Geometry check sheet. Reference: the model listing, model coordinates, mm. A direction names the side the tool comes from. Round coordinates to 2 decimals unless told otherwise and drop trailing zeros. Order: outer loops, then holes, each group sorted by start corner. A loop starts at its lowest first (then second) coordinate and runs counter-clockwise, first axis right, second up. Notation, with made-up numbers: (-16.75, -28) - (-1.75, -28) arc R15 cw to (-1.75, -15) - close; hole circle Ø3 at (-29.5, -21.75). An arc over 180 degrees is marked (long way). One line per question, with ' | ' between items. Start each with the question number.
Q1. Sectioned sample at B-B, the plane z = 67. Enter the section's corners in (x, y).
Q2. Tool access check on faces 1 (the face through (0, -356, -508)), 2 (the face through (0, 2, 584.2)). Record the directions out of +Z, -Z, +X, -X, +Y, -Y that give a thin tool (end or side, any length) a straight path to the whole face; none if there is none.
Q3. Material ranges on line 1 along Y through (x, z) = (-6, -224.5); line 2 along Z through (x, y) = (-5.25, -388.5); line 3 along Y through (x, z) = (-1, -358), recorded low to high.
Q4. Sectioned sample at C-C, the plane y = -225. Enter the section's corners in (x, z).
Q5. Sectioned sample at A-A, the plane x = -1.75. Enter the section's corners in (y, z).
Q6. Gauge pin test, flat ends, axial feed: P1, Ø12.5, axis at x = -5, z = 147, coming from the -Y side; P2, Ø12.5, axis at x = 6, y = -336, coming from the +Z side. Record the tip position at first contact, or that the pin passes through.
```python
from build123d import *

# Parameters (mm, degrees)
F0_W     = 355.6
F0_H     = 254
F1_DEPTH = 12.7
F3_DEPTH = 25.401


with BuildPart() as f1:
    # F0 (on Right) → F1 (new body, symmetric)
    with BuildSketch(Plane.YZ):
        Polygon((127, -584.2), (127, 584.2), (-127, 584.2), (-127, -330.2), (-127, -584.2), align=None)
        with Locations((-304.8, -457.2)):
            Rectangle(F0_W, F0_H)
    extrude(amount=F1_DEPTH, both=True)

    # F2 (on face) → F3 (cut, through all)
    with BuildSketch(Plane.YZ.offset(12.7)):
        with BuildLine():
            ThreePointArc((-304.8, -508), (-179.076414305, -455.923585695), (-127, -330.2))
            Line((-127, -330.2), (-482.6, -330.2))
            Line((-482.6, -330.2), (-482.6, -584.2))
            ThreePointArc((-482.6, -584.2), (-460.2815367264, -530.3184632736), (-406.4, -508))
            Line((-406.4, -508), (-304.8, -508))
        make_face()
    extrude(amount=-F3_DEPTH, mode=Mode.SUBTRACT)


solid = f1.part
```
Determined:
1) outline: (-12.7, -127) - (12.7, -127) - (12.7, 127) - (-12.7, 127) - close
2) face 1: +Z, +X, -X, -Y | face 2: +Z, +X, -X, +Y, -Y
3) line 1: y = -127 to 127 | line 2: z = -584.2 to -508 | line 3: y = -129.19 to 127
4) outline: (-12.7, -584.2) - (12.7, -584.2) - (12.7, -489.09) - (-12.7, -489.09) - close
5) outline: (-482.6, -584.2) - (127, -584.2) - (127, 584.2) - (-127, 584.2) - (-127, -330.2) arc R177.8 cw to (-304.8, -508) - (-406.4, -508) arc R76.2 ccw to start
6) P1: stops at y = -127 | P2: stops at z = -508
